Geometry check sheet. Reference: drawing and pictorial views, mm from the part's lowest x, y, z. A direction names the side the tool comes from. Coordinates: 2 decimals unless noted, no trailing zeros. Write each loop counter-clockwise with the first axis right and the second up, starting at its lowest first coordinate (ties: lowest second). Pieces come first, ordered by that corner, then holes. Notation, with made-up numbers: M 9.5,83.25 L 47.5,83.25 A20 cw 47.5,104.25 Z; hole C 72.5,25 d8. An arc over 180 degrees is marked long. One line per item, written item: value.
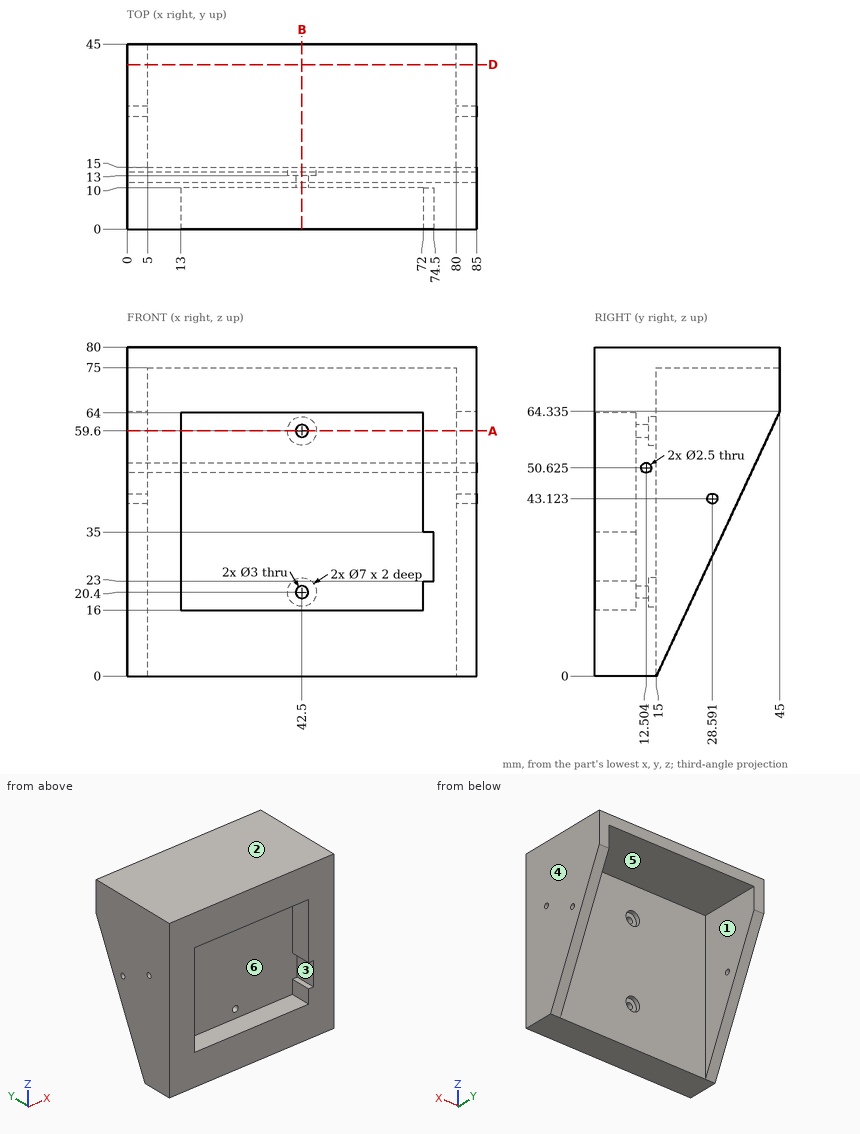
Item 1: Cross-section at A-A, the plane z = 59.6. Enter the section's corners in (x, y).
The answers:
outline: M 0,0 L 13,0 L 13,10 L 41,10 L 41,13 L 39,13 L 39,15 L 5,15 L 5,42.79 L 0,42.79 Z; M 44,10 L 72,10 L 72,0 L 85,0 L 85,42.79 L 80,42.79 L 80,15 L 46,15 L 46,13 L 44,13 Z
Item 2: Access from +Z, -Z, +X, -X, +Y, -Y to the whole of each face (thin tool, end or side, straight path). Record for the marked faces 1, 2 and 3.
The answers:
face 1: -Z, +Y
face 2: +Z, +X, -X, +Y, -Y
face 3: -Y
Item 3: Cross-section at B-B, the plane x = 42.5. Give the number of separate pieces and of enclosed holes in the cut face, and give its area (3 significant figures).
The answers:
separate pieces: 3
enclosed holes: 1
area: 819 mm²
Item 4: Go/stop test with flat-tipped pins: P1, Ø6.5, axis at x = 42.5, z = 20.4, coming from the +Y side; P2, Ø7.5, axis at x = 43, z = 19, coming from the +Y side; P3, Ø4, axis at x = 42.5, z = 59.6, coming from the -Y side. Record where each tip stops, or that it passes through.
The answers:
P1: stops at y = 13
P2: stops at y = 15
P3: stops at y = 10
Item 5: Cross-section at D-D, the plane y = 40. Enter the section's corners in (x, z).
The answers:
outline: M 0,53.61 L 5,53.61 L 5,75 L 80,75 L 80,53.61 L 85,53.61 L 85,80 L 0,80 Z
Item 6: Draft check along Z on the marked faces 4, 5 and 6. Enter one of: released by +Z, released by -Z, zero draft, split by the parting line, or undercut.
The answers:
face 4: zero draft
face 5: released by -Z
face 6: undercut
Item 7: Scan lines: line 1 (Z direction, x = 43, y = 8); line 2 (X direction, y = 42.5, z = 66); line 3 (Z direction, x = 73, y = 4). Record each from-to range of solid material in increasing order.
The answers:
line 1: z = 0 to 16, 64 to 80
line 2: x = 0 to 5, 80 to 85
line 3: z = 0 to 23, 35 to 80
